Part model, mm, in its own coordinate system. Face numbers are marked on the shaded views. A direction names the side the tool comes from. Round coordinates to 2 decimals unless told otherwise and drop trailing zeros. Order: outer loops, then holes, each group sorted by start corner. A loop starts at its lowest first (then second) coordinate and runs counter-clockwise, first axis right, second up. Notation, with made-up numbers: (52, 23) -> (81, 23) arc R27 ccw to (81, 62) -> close; hole circle Ø6 at (72.5, 41.25). An arc over 180 degrees is marked (long way). Answer as a JSON object with one key per item and string values. Group by question number.
```python
from build123d import *

# Parameters (mm, degrees)
EXTRUDE_1_DEPTH     = 270
CUT_EXTRUDE_1_REACH = 274.305
SKETCH_2_R          = 2.2


with BuildPart() as part:
    # Эскиз1 → Бобышка-Вытянуть1 (new body)
    with BuildSketch(Plane.XY):
        Polygon((0, 0), (0, -25), (1.5, -25), (1.5, -1.5), (25, -1.5), (25, 0), align=None)
    extrude(amount=EXTRUDE_1_DEPTH)

    # Эскиз2 → Вырез-Вытянуть1 (cut, up to next)
    with BuildSketch(Plane(origin=(0, 0, 0), x_dir=(1, 0, 0), z_dir=(0, 1, 0)), mode=Mode.PRIVATE) as cut_extrude_1_sk1:
        with Locations(Location((12.5, -257.5, 0), (0, 0, 270))):
            Circle(SKETCH_2_R)
    cut_extrude_1_tool1 = extrude(cut_extrude_1_sk1.sketch, amount=-CUT_EXTRUDE_1_REACH, mode=Mode.PRIVATE) & part.part
    # Эскиз2 → Вырез-Вытянуть1 (cut, up to next)
    with BuildSketch(Plane(origin=(0, 0, 0), x_dir=(1, 0, 0), z_dir=(0, 1, 0)), mode=Mode.PRIVATE) as cut_extrude_1_sk2:
        with Locations(Location((12.5, -12.5, 0), (0, 0, 270))):
            Circle(SKETCH_2_R)
    cut_extrude_1_tool2 = extrude(cut_extrude_1_sk2.sketch, amount=-CUT_EXTRUDE_1_REACH, mode=Mode.PRIVATE) & part.part
    add(cut_extrude_1_tool1.solids().sort_by_distance((12.5, 0, 257.5))[0], mode=Mode.SUBTRACT)
    add(cut_extrude_1_tool2.solids().sort_by_distance((12.5, 0, 12.5))[0], mode=Mode.SUBTRACT)


solid = part.part
```
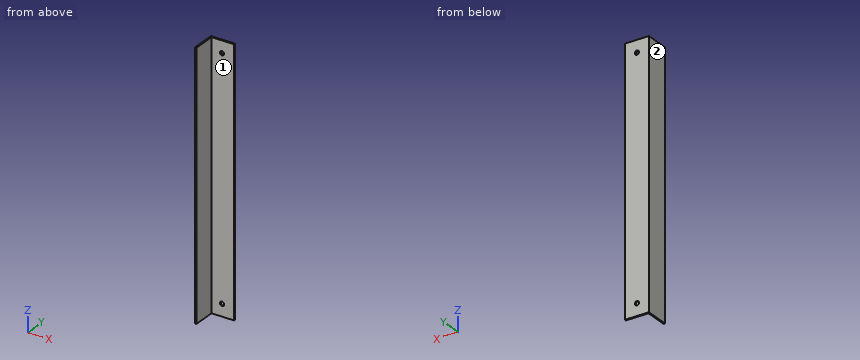
Q1. Band-saw the part on C-C (y = -6.25). List the corners of the cut face in (x, z), plus the area to 3 significant figures.
Q2. Band-saw the part on B-B (z = 257.5). List the corners of the cut face in (x, y).
Q3. Wall check: line 1 (X direction, y = -0.7, z = 257.5); line 2 (X direction, y = -11.25, z = 50); line 3 (Y direction, x = 22.75, z = 98). Give the ranges that are in metal, low to high. Write a range as [from, to].
Q4. Which spindle directions (+Z, -Z, +X, -X, +Y, -Y) get a long thin tool onto all of the face, cutting with end or side? Do the marked faces 1 and 2. Say none if no direction does.
Q5. Band-saw the part on A-A (x = 12.5). List the corners of the cut face in (y, z), plus the area to 3 significant figures.
Q6. Drop flat-ended pins along their axis: pin 1 Ø7 at (x, z) = (12.5, 257.5) entering from -Y; pin 2 Ø2.5 at (x, z) = (12.5, 12.5) entering from +Y; pin 3 Ø12 at (y, z) = (-12, 97.5) entering from +X. Give the stop position or say it passes through.
Completed:
{
 "1": {"outline": "(0, 0) -> (1.5, 0) -> (1.5, 270) -> (0, 270) -> close", "area": "405 mm2"},
 "2": {"outline": "(0, -25) -> (1.5, -25) -> (1.5, -1.5) -> (10.3, -1.5) -> (10.3, 0) -> (0, 0) -> close; (14.7, -1.5) -> (25, -1.5) -> (25, 0) -> (14.7, 0) -> close"},
 "3": {"line 1": "[0, 10.3], [14.7, 25]", "line 2": "[0, 1.5]", "line 3": "[-1.5, 0]"},
 "4": {"face 1": "+Z, -Z, +X, -Y", "face 2": "+Z, -Z, -X, +Y, -Y"},
 "5": {"outline": "(-1.5, 0) -> (0, 0) -> (0, 10.3) -> (-1.5, 10.3) -> close; (-1.5, 14.7) -> (0, 14.7) -> (0, 255.3) -> (-1.5, 255.3) -> close; (-1.5, 259.7) -> (0, 259.7) -> (0, 270) -> (-1.5, 270) -> close", "area": "392 mm2"},
 "6": {"pin 1": "y = -1.5", "pin 2": "through", "pin 3": "x = 1.5"}
}
